For this review, take the finished solid that the model builds, in its own axes (mm). A direction names the side the tool comes from. Give positions to 0.01 mm unless a question says otherwise; leave off trailing zeros. Write each loop counter-clockwise with the first axis right and the second up, starting at its lowest first coordinate (ties: lowest second). Pieces come first, ordered by that corner, then holes.
1) We need section B-B on x = 4. Give the boundary of the cut face in (y, z), and give its area (3 significant figures).
2) We need section C-C on y = 1. Give the boundary of the cut face in (x, z).
3) We need section D-D on x = 14.5. Give the boundary of the cut face in (y, z), and give its area (3 significant figures).
4) Wall thickness on line 1 along X through (y, z) = (4, 0); line 2 along X through (y, z) = (4, 7); line 3 along Z through (x, y) = (43, 0.5): over which ranges is each line inside the solid? List them lowest first.
5) Machinability: for faces 1 (the face through (22, 3, 1.75)), 2 (the face through (23, 3, -1.75)), 3 (the face through (53, 3, 3.5)), which of the approach directions +Z, -Z, +X, -X, +Y, -Y give a long, thin tool a straight path to every point of the face, cutting with its end or side? Answer none if there is none.
6) We need section A-A on z = 0. Give the boundary of the cut face in (x, y), and give its area (4 significant figures).
7) For P1, Ø0.5, axis at y = 3.5, z = 2.5, coming from the -X side; P2, Ø1, axis at y = 3.5, z = 4.5, coming from the -X side; P3, Ø1.4, axis at y = 2, z = -2.5, coming from the -X side, all flat-tipped, find the tip position at first contact; note any pin that passes through.
from build123d import *

# Parameters (mm, degrees)
SKETCH1_R           = 2.5
BOSS_EXTRUDE1_DEPTH = 7


with BuildPart() as part:
    # Sketch1 → Boss-Extrude1 (new body)
    with BuildSketch(Plane(origin=(0, 0, 0), x_dir=(1, 0, 0), z_dir=(0, 1, 0))):
        with BuildLine():
            Line((68, 3.5), (38, 3.5))
            Line((38, 3.5), (38, 1.75))
            Line((38, 1.75), (7.031088913, 1.75))
            ThreePointArc((7.031088913, 1.75), (0.5, 0), (7.031088913, -1.75))
            Line((7.031088913, -1.75), (38, -1.75))
            Line((38, -1.75), (38, -3.5))
            Line((38, -3.5), (68, -3.5))
            Line((68, -3.5), (68, -7))
            ThreePointArc((68, -7), (72, -11), (76, -7))
            Line((76, -7), (76, 3.5))
            Line((76, 3.5), (68, 3.5))
        make_face()
        with Locations(Location((72, -7, 0), (0, 0, 270))):
            Circle(SKETCH1_R, mode=Mode.SUBTRACT)
        with Locations(Location((4, 0, 0), (0, 0, 270))):
            Circle(SKETCH1_R, mode=Mode.SUBTRACT)
    extrude(amount=BOSS_EXTRUDE1_DEPTH)


solid = part.part
Results list:
1. outline: (0, -3.5) - (7, -3.5) - (7, -2.5) - (0, -2.5) - close; (0, 2.5) - (7, 2.5) - (7, 3.5) - (0, 3.5) - close
1. area: 14.0 mm2
2. outline: (7.03, -1.75) - (38, -1.75) - (38, -3.5) - (76, -3.5) - (76, 7) arc R4 ccw to (68, 7) - (68, 3.5) - (38, 3.5) - (38, 1.75) - (7.03, 1.75) arc R3.5 ccw (long way) to start; hole circle Ø5 at (4, 0); hole circle Ø5 at (72, 7)
3. outline: (0, -1.75) - (7, -1.75) - (7, 1.75) - (0, 1.75) - close
3. area: 24.5 mm2
4. line 1: x = 0.5 to 1.5, 6.5 to 76
4. line 2: x = 68 to 69.5, 74.5 to 76
4. line 3: z = -3.5 to 3.5
5. face 1: +Z, +Y, -Y
5. face 2: -Z, +Y, -Y
5. face 3: +Z, -X, +Y, -Y
6. outline: (0.5, 0) - (1.5, 0) - (1.5, 7) - (0.5, 7) - close; (6.5, 0) - (76, 0) - (76, 7) - (6.5, 7) - close
6. area: 493.5 mm2
7. P1: stops at x = 1.32
7. P2: stops at x = 68
7. P3: stops at x = 1
